from build123d import *

# Parameters (mm, degrees)
F0_W      = 96.0585176945
F0_H      = 59.3097396195
F1_DEPTH  = 25.4
F2_R      = 6.9698590231
F3_DEPTH  = 25.4
F4_R      = 8.3090946214
F5_DEPTH  = 43.688
F7_DEPTH  = 28.702
F9_DEPTH  = 25.4
F11_DEPTH = 36.83


with BuildPart() as f1:
    # F0 (on Top) → F1 (new body)
    with BuildSketch(Plane.XY):
        with Locations((23.4913080931, 1.3955235481)):
            Rectangle(F0_W, F0_H)
        with BuildLine():
            Line((-24.5379507542, -28.2593462616), (-24.5379507542, 31.0503933579))
            ThreePointArc((-24.5379507542, 31.0503933579), (-70.8578223618, 1.3955235481), (-24.5379507542, -28.2593462616))
        make_face()
    extrude(amount=F1_DEPTH)

    # F2 (on Top) → F3 (join)
    with BuildSketch(Plane.XY):
        with Locations((-53.8439378142, 0)):
            Circle(F2_R)
    extrude(amount=F3_DEPTH)

    # F4 (on Top) → F5 (cut)
    with BuildSketch(Plane.XY):
        with Locations((-59.1934472322, 0)):
            Circle(F4_R)
    extrude(amount=F5_DEPTH, mode=Mode.SUBTRACT)

    # F6 (on Top) → F7 (cut)
    with BuildSketch(Plane.XY):
        with BuildLine():
            add(Edge.make_bspline(
                [(-2.1032807417, 46.1836736649), (-12.042039887, 46.1836736649), (-7.0726603144, 23.6138207838), (-2.1032807417, 1.0439679027), (2.8660988309, 23.6138207838), (7.8354784036, 46.1836736649), (-2.1032807417, 46.1836736649)],
                knots=[0, 0, 0, 2.0943951024, 2.0943951024, 4.1887902048, 4.1887902048, 6.2831853072, 6.2831853072, 6.2831853072], degree=2, weights=[1, 0.5, 1, 0.5, 1, 0.5, 1]))
        make_face()
        with BuildLine():
            add(Edge.make_bspline(
                [(13.6858932674, 41.4513960598), (6.7221471859, 41.4513960598), (10.2040202267, 25.6374778168), (13.6858932674, 9.8235595737), (17.1677663081, 25.6374778168), (20.6496393489, 41.4513960598), (13.6858932674, 41.4513960598)],
                knots=[0, 0, 0, 2.0943951024, 2.0943951024, 4.1887902048, 4.1887902048, 6.2831853072, 6.2831853072, 6.2831853072], degree=2, weights=[1, 0.5, 1, 0.5, 1, 0.5, 1]))
        make_face()
        with BuildLine():
            add(Edge.make_bspline(
                [(29.2345341295, 46.4820731431), (19.2957749842, 46.4820731431), (24.2651545569, 23.912220262), (29.2345341295, 1.3423673809), (34.2039137021, 23.912220262), (39.1732932748, 46.4820731431), (29.2345341295, 46.4820731431)],
                knots=[0, 0, 0, 2.0943951024, 2.0943951024, 4.1887902048, 4.1887902048, 6.2831853072, 6.2831853072, 6.2831853072], degree=2, weights=[1, 0.5, 1, 0.5, 1, 0.5, 1]))
        make_face()
        with BuildLine():
            add(Edge.make_bspline(
                [(45.7755737007, 41.7389214156), (38.8118276192, 41.7389214156), (42.2937006599, 25.9250031726), (45.7755737007, 10.1110849296), (49.2574467414, 25.9250031726), (52.7393197821, 41.7389214156), (45.7755737007, 41.7389214156)],
                knots=[0, 0, 0, 2.0943951024, 2.0943951024, 4.1887902048, 4.1887902048, 6.2831853072, 6.2831853072, 6.2831853072], degree=2, weights=[1, 0.5, 1, 0.5, 1, 0.5, 1]))
        make_face()
        with BuildLine():
            add(Edge.make_bspline(
                [(60.8162461653, 46.2759053466), (50.87748702, 46.2759053466), (55.8468665926, 23.7060524655), (60.8162461653, 1.1361995844), (65.7856257379, 23.7060524655), (70.7550053106, 46.2759053466), (60.8162461653, 46.2759053466)],
                knots=[0, 0, 0, 2.0943951024, 2.0943951024, 4.1887902048, 4.1887902048, 6.2831853072, 6.2831853072, 6.2831853072], degree=2, weights=[1, 0.5, 1, 0.5, 1, 0.5, 1]))
        make_face()
    extrude(amount=F7_DEPTH, mode=Mode.SUBTRACT)

    # F8 (on Top) → F9 (cut)
    with BuildSketch(Plane.XY):
        Polygon((71.7460587621, -22.2876053303), (-17.4043662846, -22.2876053303), (-17.4043662846, -27.296056971), (-17.4043662846, -33.5566177964), (71.7460587621, -33.5566177964), align=None)
    extrude(amount=-F9_DEPTH, mode=Mode.SUBTRACT)

    # F10 (on Top) → F11 (cut)
    with BuildSketch(Plane.XY):
        Polygon((-23.9153504372, -25.2926759422), (-23.6649308354, -35.5600006878), (-12.1454931796, -35.5600006878), (-12.1454931796, -25.2926759422), align=None)
    extrude(amount=F11_DEPTH, mode=Mode.SUBTRACT)


solid = f1.part
Design review of the part built by this model. Coordinates are the model's own, in mm. A direction names the side the tool comes from. Give positions to 0.01 mm unless a question says otherwise; leave off trailing zeros. Loops run counter-clockwise (first coordinate to the right, second up) from the corner with the lowest first, then second, coordinate; pieces in that order, holes last. Notation, with made-up numbers: (9, -5) - (32, -5) arc R19 cw to (32, 22) - close; hole circle Ø2 at (-29.75, -21). An arc over 180 degrees is marked (long way). Use CSV: the item, a comma, the result in double quotes. Start each with the question number.
1. Add section B-B (y = 0). State the section outline as (x, z) points, plus the area to 3 significant figures.
2. Machinability: for faces 5 (the flat face through (29, -28.259, 13)), 6 (the flat face through (38, 31.05, 13)), 7 (the flat face through (-12.145, -27, 13)), which of the approach directions +Z, -Z, +X, -X, +Y, -Y give a long, thin tool a straight path to every point of the face, cutting with its end or side? Answer none if there is none.
3. Wall thickness on L1, parallel to X at y = 27.5, z = 13.25; L2, parallel to Y at x = 38, z = 21: over which ranges is each line inside the solid? List them lowest first.
4. Draft analysis for pull direction X (two halves, no side actions). For faces 1 (the flat face through (21, 31.05, 13)), 2 (the flat face through (-18, -25.293, 13)), 3 (the flat face through (71.521, 1, 13)), 4 (the cylindrical face through (-70.845, 2.311, 12.522)), state which applies: released by +X, released by -X, zero draft, split by the parting line, or undercut.
5. Insertion check: P1, Ø2.5, axis at x = 51.5, z = 19, coming from the +Y side; P2, Ø2, axis at y = 6.5, z = 12, coming from the -X side; P3, Ø1, axis at x = 19.5, z = 5.5, coming from the -Y side; P4, Ø3, axis at x = -1.5, y = 19.5, coming from the -Z side. Each pin has a flat end and moves straight along its axis. Give the tip position at first contact, or say it passes through.
6. Add section A-A (x = -60). State the section outline as (y, z) points.
7. Add section C-C (x = -29.5). State the section outline as (y, z) points, plus the area to 3 significant figures.
8. Add section D-D (y = -21). State the section outline as (x, z) points, plus the area to 3 significant figures.
Results found:
1,outline,"(-70.83, 0) - (-67.5, 0) - (-67.5, 25.4) - (-70.83, 25.4) - close; (-50.88, 0) - (71.52, 0) - (71.52, 25.4) - (-50.88, 25.4) - close"
1,area,"3,190 mm²"
2,face 5,"+Z, -Z, +X, -Y"
2,face 6,"+Z, -Z, +X, +Y"
2,face 7,"+Z, -Z, -Y"
3,L1,"x = -57.82 to -7.67, 3.46 to 9.88, 17.49 to 23.7, 34.77 to 42.01, 49.54 to 55.26, 66.38 to 71.52"
3,L2,"y = -28.26 to 31.05"
4,face 1,"zero draft"
4,face 2,"undercut"
4,face 3,"released by +X"
4,face 4,"split by the parting line"
5,P1,"stops at y = 31.05"
5,P2,"stops at x = -70.6"
5,P3,"stops at y = -28.26"
5,P4,"passes through"
6,outline,"(-22.92, 0) - (-8.27, 0) - (-8.27, 25.4) - (-22.92, 25.4) - close; (8.27, 0) - (25.71, 0) - (25.71, 25.4) - (8.27, 25.4) - close"
7,outline,"(-30.08, 0) - (32.87, 0) - (32.87, 25.4) - (-30.08, 25.4) - close"
7,area,"1,600 mm²"
8,outline,"(-61.97, 0) - (71.52, 0) - (71.52, 25.4) - (-61.97, 25.4) - close"
8,area,"3,390 mm²"
